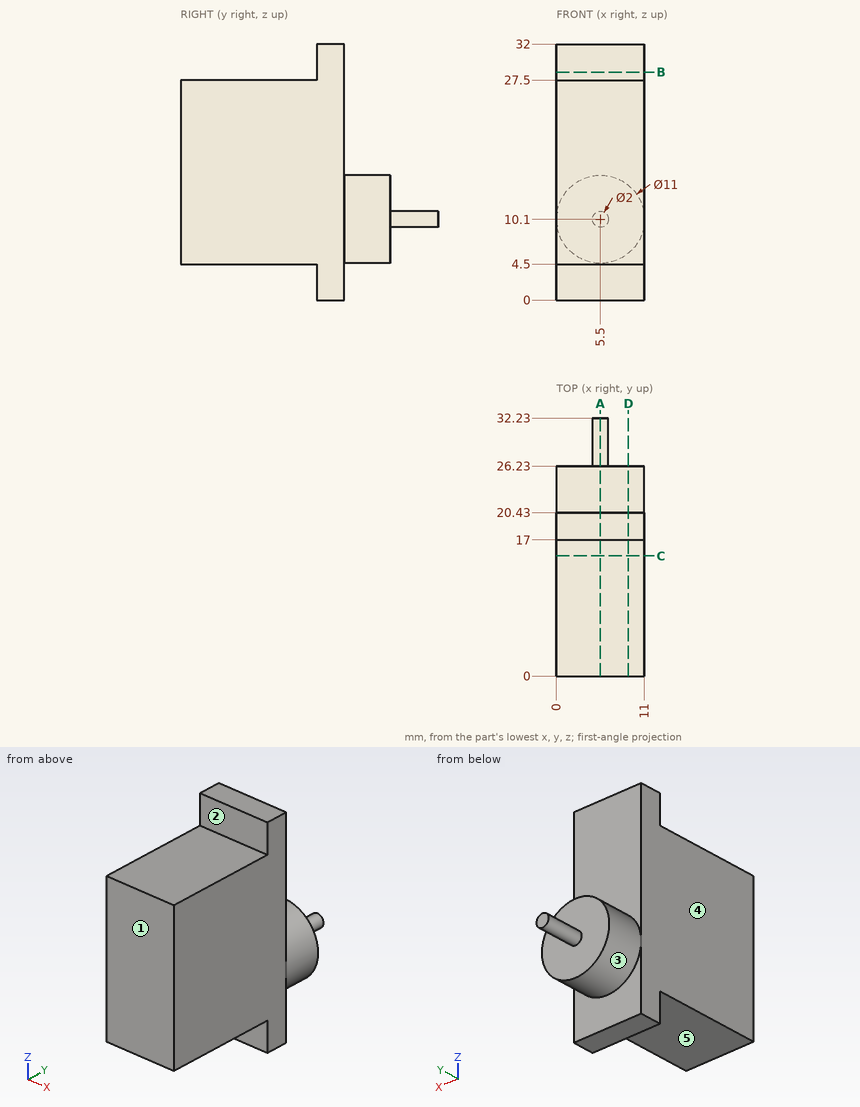
Source: three-view drawing plus pictorial views. Frame: mm from the lowest corner of the part. A direction names the side the tool comes from. Coordinates: 2 decimals unless noted, no trailing zeros. Order: outer loops, then holes, each group sorted by start corner. A loop starts at its lowest first (then second) coordinate and runs counter-clockwise, first axis right, second up.
1) Section B-B (z = 28.5). Return loops of the section in (x, y), then the cut area to 3 significant figures.
Result sheet:
outline: (0, 17) - (11, 17) - (11, 20.43) - (0, 20.43) - close
area: 37.7 mm2
2) Section A-A (x = 5.5). Return loops of the section in (y, z), then the cut area to 3 significant figures.
Result sheet:
outline: (0, 4.5) - (17, 4.5) - (17, 0) - (20.43, 0) - (20.43, 4.6) - (26.23, 4.6) - (26.23, 9.1) - (32.23, 9.1) - (32.23, 11.1) - (26.23, 11.1) - (26.23, 15.6) - (20.43, 15.6) - (20.43, 32) - (17, 32) - (17, 27.5) - (0, 27.5) - close
area: 577 mm2
3) First-contact query: P1, Ø2, axis at x = 2, y = 25.5, coming from the +Z side; P2, Ø2, axis at x = 3, z = 2.5, coming from the -Y side; P3, Ø5.5, axis at x = 8, y = 5, coming from the -Z side. Flat tips, straight axial feed; report the tip coordinate or a pass-through.
Result sheet:
P1: stops at z = 15
P2: stops at y = 17
P3: stops at z = 4.5
4) Ray query, probe 1 along Y at (x, z) = (9.25, 25); probe 2 along Y at (x, z) = (7.75, 14.5); probe 3 along Z at (x, y) = (2, 10). Return the intervals inside material, ascending.
Result sheet:
probe 1: y = 0 to 20.43
probe 2: y = 0 to 26.23
probe 3: z = 4.5 to 27.5
5) Section D-D (x = 9). Return loops of the section in (y, z), then the cut area to 3 significant figures.
Result sheet:
outline: (0, 4.5) - (17, 4.5) - (17, 0) - (20.43, 0) - (20.43, 5.86) - (26.23, 5.86) - (26.23, 14.34) - (20.43, 14.34) - (20.43, 32) - (17, 32) - (17, 27.5) - (0, 27.5) - close
area: 550 mm2
6) Set-up query: the marked faces 1, 2, 3, 4 and 5. Return all of +Z, -Z, +X, -X, +Y, -Y with unobstructed straight access to the full face (end or side cutting, diameter ignored); none if empty.
Result sheet:
face 1: +Z, -Z, +X, -X, -Y
face 2: +Z, +X, -X, -Y
face 3: +Y
face 4: +Z, -Z, -X, +Y, -Y
face 5: -Z, +X, -X, -Y
7) Section C-C (y = 15). Return loops of the section in (x, z), then the cut area to 3 significant figures.
Result sheet:
outline: (0, 4.5) - (11, 4.5) - (11, 27.5) - (0, 27.5) - close
area: 253 mm2
